Can you work these out from the model? Positions are in its coordinate system, mm. A direction names the side the tool comes from. Give positions to 0.01 mm unless a question says otherwise; leave off trailing zeros. Order: outer loops, then holes, each group sorted by start corner. A loop starts at its lowest first (then second) coordinate and runs counter-clockwise, first axis right, second up. Notation, with made-up numbers: M -3,31 L 27,31 A12 ccw 27,44 Z; hole C 39.25,18 d2. An arc over 180 degrees is marked long. Use one line per item in the form item = value. Start each with the question number.
1. I want a section at C-C, the plane y = 2. List the corners of the cut face in (x, z) for me, and give its area (3 significant figures).
2. I want a section at B-B, the plane z = -5.5. List the corners of the cut face in (x, y) for me, and give its area (3 significant figures).
3. I want a section at D-D, the plane x = 3.5. List the corners of the cut face in (y, z) for me, and give its area (3 significant figures).
4. For faces 1 (the face through (6, 3, -2)), 2 (the face through (0, 2, -6)), which set-ups out of +Z, -Z, +X, -X, +Y, -Y let a thin tool reach every point of the face, with its end or its side?
5. I want a section at A-A, the plane x = 6.5. List the corners of the cut face in (y, z) for me.
6. I need wall thicknesses on L1, parallel to Y at x = 6, z = -3; L2, parallel to Y at x = 5.25, z = -4.5; L3, parallel to Z at x = 3.75, y = 1.2. Which ranges of each line are inside material? Lowest first, please.
```python
from build123d import *

# Parameters (mm, degrees)
EXTRUDE_1_DEPTH     = 4
SKETCH_2_R          = 1
CUT_EXTRUDE_1_DEPTH = 13
CUT_EXTRUDE_2_DEPTH = 13


with BuildPart() as part:
    # Эскиз1 → Бобышка-Вытянуть1 (new body)
    with BuildSketch(Plane(origin=(0, 0, 0), x_dir=(1, 0, 0), z_dir=(0, 1, 0))):
        Polygon((0, 0), (0, 12), (3.085955121, 12), (8.428699344, 0), align=None)
    extrude(amount=EXTRUDE_1_DEPTH)

    # Эскиз2 → Вырез-Вытянуть1 (cut, through all)
    with BuildSketch(Plane.XY):
        with Locations((5.7, 2)):
            Circle(SKETCH_2_R)
    extrude(amount=-CUT_EXTRUDE_1_DEPTH, mode=Mode.SUBTRACT)

    # Эскиз3 → Вырез-Вытянуть2 (cut, through all)
    with BuildSketch(Plane.XY):
        with BuildLine():
            Line((8.428699344, 3), (5.7, 3))
            ThreePointArc((5.7, 3), (6.407106781, 2.707106781), (6.7, 2))
            ThreePointArc((6.7, 2), (6.407106781, 1.292893219), (5.7, 1))
            Line((5.7, 1), (8.428699344, 1))
            Line((8.428699344, 1), (8.428699344, 3))
        make_face()
    extrude(amount=-CUT_EXTRUDE_2_DEPTH, mode=Mode.SUBTRACT)


solid = part.part
```
Check result:
q1.outline = M 0,-12 L 3.09,-12 L 4.7,-8.37 L 4.7,0 L 0,0 Z
q1.area = 53.5 mm2
q2.outline = M 0,0 L 5.98,0 L 5.98,1 L 5.7,1 A1 cw 5.7,3 L 5.98,3 L 5.98,4 L 0,4 Z
q2.area = 21.8 mm2
q3.outline = M 0,-11.07 L 4,-11.07 L 4,0 L 0,0 Z
q3.area = 44.3 mm2
q4.face_1 = +Z, -Z, +X
q4.face_2 = +Z, -Z, -X, +Y, -Y
q5.outline = M 0,-4.33 L 1,-4.33 L 1,0 L 0,0 Z; M 3,-4.33 L 4,-4.33 L 4,0 L 3,0 Z
q6.L1 = 0 to 1, 3 to 4
q6.L2 = 0 to 1.11, 2.89 to 4
q6.L3 = -10.51 to 0
